Design review of the part shown in the three views and the two pictorial views. Dimensions are in mm from the part's minimum x, y and z. A direction names the side the tool comes from. Coordinates: 2 decimals unless noted, no trailing zeros. Loops run counter-clockwise (first coordinate to the right, second up) from the corner with the lowest first, then second, coordinate; pieces in that order, holes last. Notation, with made-up numbers: M 6.5,-32.75 L 21.5,-32.75 A28 ccw 21.5,-2.75 Z; hole C 59,28.25 d4. An arc over 180 degrees is marked long. Write item = value, one per line. Start each with the question number.
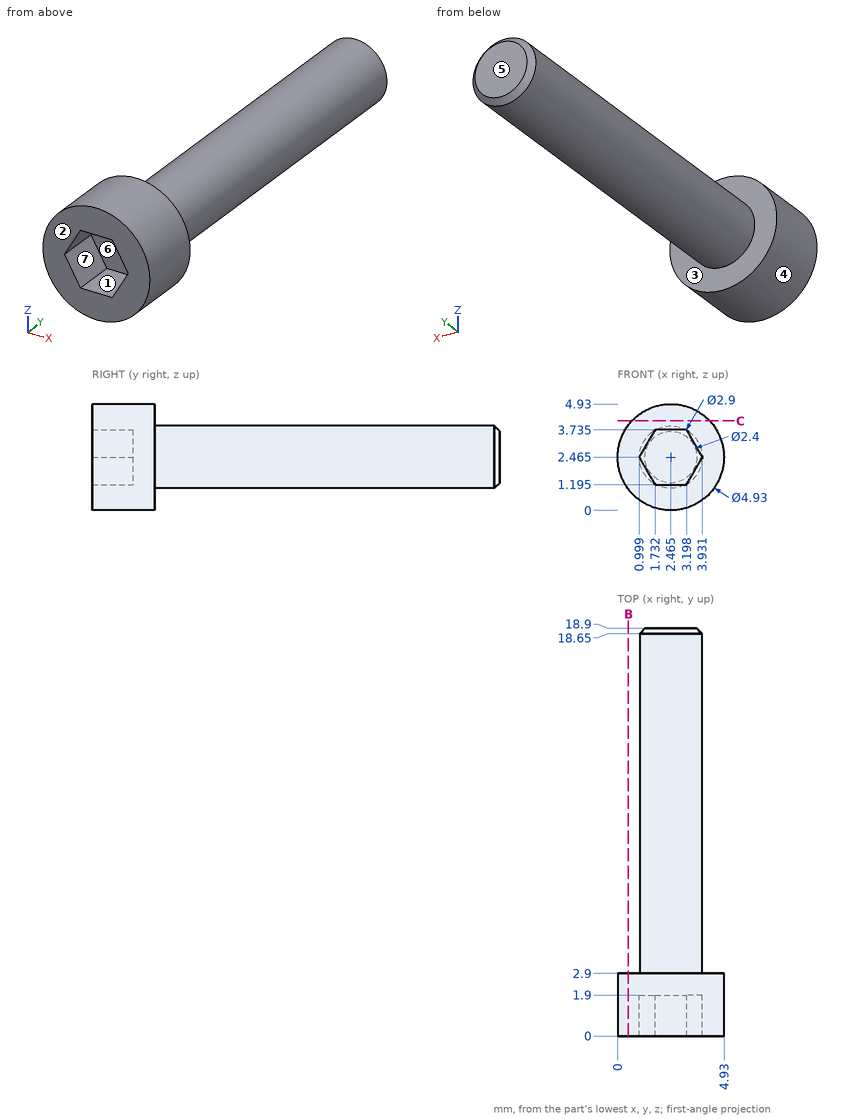
(1) To check wall thickness, follow L1, parallel to Z at x = 2.6, y = 1.25 (1 decimal); L2, parallel to Y at x = 2, z = 0.95; L3, parallel to Y at x = 2.1, z = 2.7. State the ranges of each line that lie inside material, in increasing order.
(2) Mouldability with a two-part tool opening along Z and no side actions: class the marked faces 4, 5, 6 and 7 as +Z half, -Z half, draft (parallel to the pull), parting line (faces both ways), or undercut.
(3) Insertion check: pin 1 (0.8 mm diameter, centred on x = 2.5, z = 2.5, fed in from -Y); pin 2 (2 mm diameter, centred on y = 16, z = 3.5, fed in from +X) (1 decimal); pin 3 (1 mm diameter, centred on x = 3, y = 3.5, fed in from +Z) (1 decimal). Each pin has a flat end and moves straight along its axis. Give the tip position at first contact, or say it passes through.
(4) Take a section at C-C (z = 4.15). State the section outline as (x, y) points (1 decimal).
(5) Tool access review of the marked faces 1, 2 and 3: name each direction out of +Z, -Z, +X, -X, +Y, -Y from which nothing blocks a thin tool from reaching the whole face with its end or side.
(6) Take a section at B-B (x = 0.5). State the section outline as (y, z) points.
Results list:
q1.L1 = 0 to 1.2, 3.7 to 4.9
q1.L2 = 0 to 2.9
q1.L3 = 1.9 to 18.9
q2.face_4 = parting line
q2.face_5 = draft
q2.face_6 = undercut
q2.face_7 = undercut
q3.pin_1 = 1.9
q3.pin_2 = 3.9
q3.pin_3 = 3.9
q4.outline = M 0.7,0 L 4.3,0 L 4.3,2.9 L 0.7,2.9 Z
q5.face_1 = -Y
q5.face_2 = +Z, -Z, +X, -X, -Y
q5.face_3 = +Y
q6.outline = M 0,0.98 L 2.9,0.98 L 2.9,3.95 L 0,3.95 Z
